```python
from build123d import *

# Parameters (mm, degrees)
SKETCH1_R                 = 4.7625
BOSS_EXTRUDE1_DEPTH       = 10.09015
CUT_EXTRUDE1_DEPTH        = 13.49375
CUT_EXTRUDE1_DEPTH_BACK   = 13.49375
SKETCH2_W                 = 3.175
SKETCH2_H                 = 3.175
SKETCH2_W_2               = 0.335237521
SKETCH2_H_2               = 0.139682301
F_4_40_TAPPED_HOLE1_D     = 2.2606
F_4_40_TAPPED_HOLE1_DEPTH = 8.8646
F_4_40_TAPPED_HOLE1_TIP   = 0.679152758
SKETCH6_R                 = 6.35
BOSS_EXTRUDE2_DEPTH       = 1.27


with BuildPart() as part:
    # Sketch1 → Boss-Extrude1 (new body)
    with BuildSketch(Plane.XY):
        Circle(SKETCH1_R)
    extrude(amount=BOSS_EXTRUDE1_DEPTH)

    # Sketch2 → Cut-Extrude1 (cut, two sides: drawn at the far end of the back side and taken through both)
    with BuildSketch(Plane(origin=(0, 0, 0), x_dir=(1, 0, 0), z_dir=(0, 1, 0)).offset(-CUT_EXTRUDE1_DEPTH_BACK)):
        with Locations((-3.175, -1.1303)):
            Rectangle(SKETCH2_W, SKETCH2_H)
        with Locations((6.06221185, 0.404858795)):
            Rectangle(SKETCH2_W_2, SKETCH2_H_2)
        with Locations((3.175, -1.1303)):
            Rectangle(SKETCH2_W, SKETCH2_H)
    extrude(amount=CUT_EXTRUDE1_DEPTH + CUT_EXTRUDE1_DEPTH_BACK, mode=Mode.SUBTRACT)

    # #4-40 Tapped Hole1
    with Locations(Plane(origin=(0, 0, 0), x_dir=(-1, 0, 0), z_dir=(0, 0, -1))):
        with Locations((0, 0)):
            Hole(F_4_40_TAPPED_HOLE1_D / 2, depth=F_4_40_TAPPED_HOLE1_DEPTH)
            with Locations((0, 0, -(F_4_40_TAPPED_HOLE1_DEPTH + F_4_40_TAPPED_HOLE1_TIP / 2))):  # 118° drill point
                Cone(0, F_4_40_TAPPED_HOLE1_D / 2, F_4_40_TAPPED_HOLE1_TIP, mode=Mode.SUBTRACT)

    # Sketch6 → Boss-Extrude2 (add)
    with BuildSketch(Plane.XY.offset(10.09015)):
        Circle(SKETCH6_R)
    extrude(amount=-BOSS_EXTRUDE2_DEPTH)


solid = part.part
```
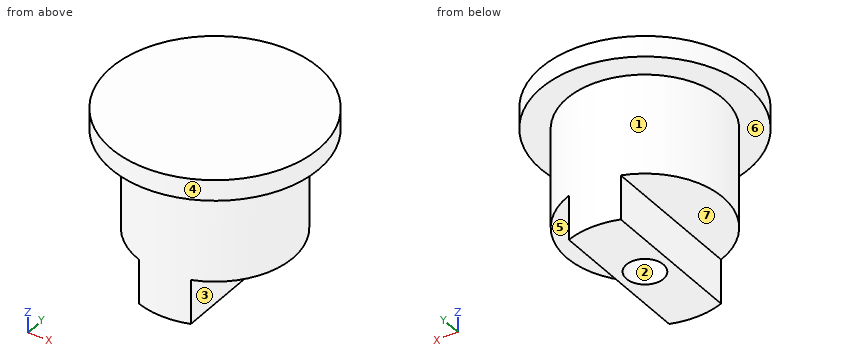
CAD build for the part. Positions are in the model's coordinates, mm. Face numbers are marked on the shaded views. A direction names the side the tool comes from. Give positions to 0.01 mm unless a question says otherwise; leave off trailing zeros. Order: outer loops, then holes, each group sorted by start corner. A loop starts at its lowest first (then second) coordinate and runs counter-clockwise, first axis right, second up. Notation, with made-up numbers: M 5.5,23 L 10.5,23 A18 ccw 10.5,35 Z; hole C 84,11.5 d1. An arc over 180 degrees is marked long. Put each result on its own line as item: value. Start each with the question number.
(1) Saw through at B-B, the plane x = 0. Write the cut outline in (y, z).
(2) Which spindle directions (+Z, -Z, +X, -X, +Y, -Y) get a long thin tool onto all of the face, cutting with end or side? Do the marked faces 4, 5, 6 and 7. Say none if no direction does.
(3) Saw through at C-C, the plane z = 7.75. Write the cut outline in (x, y) (1 decimal), then the cut area to 3 significant figures.
(4) Saw through at D-D, the plane x = -3. Write the cut outline in (y, z), then the cut area to 3 significant figures.
(5) Mould opens along Y. For the marked faces 1, 2 and 3 say: +Y half, -Y half, draft (parallel to the pull), parting line (faces both ways), or undercut.
(6) Drill centre lines: line 1 along Y through (x, z) = (0, 4.75); line 2 along Z through (x, y) = (-3.5, -2.25); line 3 along X through (y, z) = (3.25, 1.25). Where is each one in solid material? Low to high.
(7) Flat gauge pins, fed straight in: pin 1 Ø3 at (y, z) = (1.5, 1) entering from +X; pin 2 Ø2 at (x, z) = (0, 3.5) entering from +Y; pin 3 Ø1 at (x, y) = (3.5, -1) entering from -Z. Where does each tip first touch, or does it go through?
(8) Saw through at A-A, the plane y = 0. Write the cut outline in (x, z).
Check result:
1. outline: M -6.35,8.82 L -4.76,8.82 L -4.76,0 L -1.13,0 L -1.13,8.82 L 1.13,8.82 L 1.13,0 L 4.76,0 L 4.76,8.82 L 6.35,8.82 L 6.35,10.09 L -6.35,10.09 Z
2. face 4: +Z, -Z
2. face 5: -Z, +X, +Y, -Y
2. face 6: -Z
2. face 7: -Z, -X, +Y, -Y
3. outline: C 0,0 d9.5; hole C 0,0 d2.3
3. area: 67.2 mm2
4. outline: M -5.6,8.82 L -3.7,8.82 L -3.7,2.72 L 3.7,2.72 L 3.7,8.82 L 5.6,8.82 L 5.6,10.09 L -5.6,10.09 Z
4. area: 59.4 mm2
5. face 1: parting line
5. face 2: undercut
5. face 3: draft
6. line 1: y = -4.76 to -1.13, 1.13 to 4.76
6. line 2: z = 2.72 to 10.09
6. line 3: x = -1.59 to 1.59
7. pin 1: stops at x = 1.59
7. pin 2: stops at y = 4.76
7. pin 3: stops at z = 2.72
8. outline: M -6.35,8.82 L -4.76,8.82 L -4.76,2.72 L -1.59,2.72 L -1.59,0 L -1.13,0 L -1.13,8.82 L 1.13,8.82 L 1.13,0 L 1.59,0 L 1.59,2.72 L 4.76,2.72 L 4.76,8.82 L 6.35,8.82 L 6.35,10.09 L -6.35,10.09 Z
